```python
from build123d import *

# Parameters (mm, degrees)
SKETCH1_R                                           = 101.6
BOSS_EXTRUDE1_DEPTH                                 = 12.7
CSK_FOR_1_4_FLAT_HEAD_MACHINE_SCREW_100_D           = 6.7564
CSK_FOR_1_4_FLAT_HEAD_MACHINE_SCREW_100_DEPTH       = 25.4
CSK_FOR_1_4_FLAT_HEAD_MACHINE_SCREW_100_CSINK_D     = 12.8778
CSK_FOR_1_4_FLAT_HEAD_MACHINE_SCREW_100_CSINK_ANGLE = 100
CSK_FOR_1_4_FLAT_HEAD_MACHINE_SCREW_100_TIP         = 2.029827343


with BuildPart() as part:
    # Sketch1 → Boss-Extrude1 (new body)
    with BuildSketch(Plane.XY):
        Circle(SKETCH1_R)
    extrude(amount=BOSS_EXTRUDE1_DEPTH)

    # CSK for 1/4 Flat Head Machine Screw (100)1
    with Locations(Plane(origin=(0, 0, 0), x_dir=(-1, 0, 0), z_dir=(0, 0, -1))):
        with Locations((-15.875, -38.1), (-15.875, 38.1), (15.875, 38.1), (15.875, -38.1)):
            CounterSinkHole(CSK_FOR_1_4_FLAT_HEAD_MACHINE_SCREW_100_D / 2, CSK_FOR_1_4_FLAT_HEAD_MACHINE_SCREW_100_CSINK_D / 2, depth=CSK_FOR_1_4_FLAT_HEAD_MACHINE_SCREW_100_DEPTH, counter_sink_angle=CSK_FOR_1_4_FLAT_HEAD_MACHINE_SCREW_100_CSINK_ANGLE)
            with Locations((0, 0, -(CSK_FOR_1_4_FLAT_HEAD_MACHINE_SCREW_100_DEPTH + CSK_FOR_1_4_FLAT_HEAD_MACHINE_SCREW_100_TIP / 2))):  # 118° drill point
                Cone(0, CSK_FOR_1_4_FLAT_HEAD_MACHINE_SCREW_100_D / 2, CSK_FOR_1_4_FLAT_HEAD_MACHINE_SCREW_100_TIP, mode=Mode.SUBTRACT)


solid = part.part
```
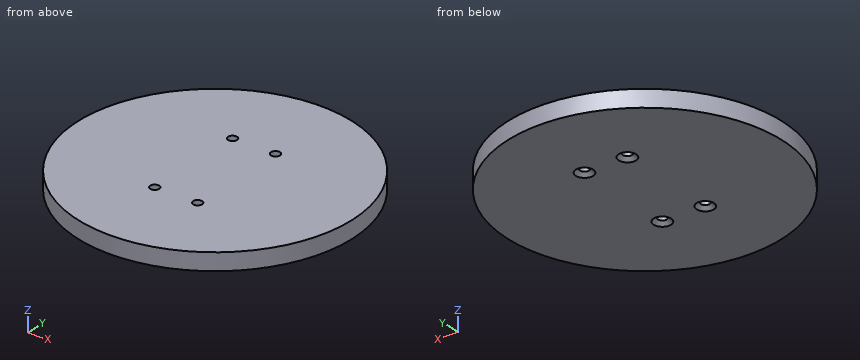
Design review of the part built by this model. Coordinates are the model's own, in mm. Round coordinates to 2 decimals unless told otherwise and drop trailing zeros. Order: outer loops, then holes, each group sorted by start corner. A loop starts at its lowest first (then second) coordinate and runs counter-clockwise, first axis right, second up. Notation, with made-up numbers: (32.5, 74) - (38.5, 74) arc R21 cw to (38.5, 103) - close; hole circle Ø11 at (7, 6). An arc over 180 degrees is marked (long way). Return JSON: item names as keys, results as strings.
Q1. Wall thickness on L1, parallel to Y at x = 13.5, z = 6.25; L2, parallel to X at y = 38.1, z = 6.75; L3, parallel to Y at x = -12, z = 1: over which ranges is each line inside the solid? List them lowest first. Write a range as [from, to].
Computed values:
{"L1": "y = [-100.7, -40.5], [-35.7, 35.7], [40.5, 100.7]", "L2": "x = [-94.19, -19.25], [-12.5, 12.5], [19.25, 94.19]", "L3": "y = [-100.89, -41.64], [-34.56, 34.56], [41.64, 100.89]"}
Q2. Consider section A-A on z = 10.5. Write out the cut boundary in (x, y) (3 decimals), plus the area to 3 significant figures.
Computed values:
{"outline": "circle Ø203.2 at (0, 0); hole circle Ø6.756 at (-15.875, -38.1); hole circle Ø6.756 at (-15.875, 38.1); hole circle Ø6.756 at (15.875, -38.1); hole circle Ø6.756 at (15.875, 38.1)", "area": "32,300 mm2"}
Q3. Consider section B-B on y = 38.1. Write out the cut boundary in (x, z), plus the area to 3 significant figures.
Computed values:
{"outline": "(-94.19, 0) - (-22.31, 0) - (-19.25, 2.57) - (-19.25, 12.7) - (-94.19, 12.7) - close; (-12.5, 2.57) - (-9.44, 0) - (9.44, 0) - (12.5, 2.57) - (12.5, 12.7) - (-12.5, 12.7) - close; (19.25, 2.57) - (22.31, 0) - (94.19, 0) - (94.19, 12.7) - (19.25, 12.7) - close", "area": "2,200 mm2"}
Q4. Consider section C-C on x = -41. Write out the cut boundary in (y, z), plus the area to 3 significant figures.
Computed values:
{"outline": "(-92.96, 0) - (92.96, 0) - (92.96, 12.7) - (-92.96, 12.7) - close", "area": "2,360 mm2"}
Q5. Consider section D-D on y = -54.5. Write out the cut boundary in (x, z).
Computed values:
{"outline": "(-85.75, 0) - (85.75, 0) - (85.75, 12.7) - (-85.75, 12.7) - close"}
Q6. For pin 1 Ø6 at (x, y) = (-15.875, -38.1) entering from +Z; pin 2 Ø4 at (x, z) = (-77.5, 5) entering from -Y; pin 3 Ø3 at (x, z) = (-5.5, 10) entering from -Y; pin 4 Ø1 at (x, z) = (62, 1.5) entering from +Y, all flat-tipped, find the tip position at first contact; note any pin that passes through.
Computed values:
{"pin 1": "passes through", "pin 2": "stops at y = -67.99", "pin 3": "stops at y = -101.52", "pin 4": "stops at y = 80.87"}
